Work out the finished part from the listing and answer in its coordinate system (mm). A direction names the side the tool comes from. Round coordinates to 2 decimals unless told otherwise and drop trailing zeros. Answer in a Markdown table with one row per item.
Autodesk Fusion 360 part; units mm, degrees
ref_plane "WorkPlane1" through (0, 0, 40) normal (0, 0, 1) x (1, 0, 0)
ref_plane "WorkPlane2" through (0, 0, 50) normal (0, 0, 1) x (1, 0, 0)
sketch "Sketch1" plane through (0, 0, 0) normal (0, 0, 1) x (1, 0, 0)
  line L0 (-21, 4) -> (119, 4)
  line L1 (119, 4) -> (119, 94)
  line L2 (119, 94) -> (-21, 94)
  line L3 (-21, 94) -> (-21, 4)
sketch "Sketch2" plane through (0, 0, 40) normal (0, 0, 1) x (1, 0, 0)
  line L0 (-1, -1) -> (99, -1)
  line L1 (99, -1) -> (99, 99)
  line L2 (99, 99) -> (-1, 99)
  line L3 (-1, 99) -> (-1, -1)
sketch "Sketch3" plane through (0, 0, 50) normal (0, 0, 1) x (1, 0, 0)
  line L0 (-1, -1) -> (99, -1)
  line L1 (99, -1) -> (99, 99)
  line L2 (99, 99) -> (-1, 99)
  line L3 (-1, 99) -> (-1, -1)
loft "Loft1" add profiles "Sketch1", "Sketch2", "Sketch3" section 1 section 2 section 3
sketch "Sketch4" plane through (0, 0, 0) normal (0, 0, 1) x (1, 0, 0)
  line L0 (-19, 6) -> (117, 6)
  line L1 (117, 6) -> (117, 92)
  line L2 (117, 92) -> (-19, 92)
  line L3 (-19, 92) -> (-19, 6)
sketch "Sketch5" plane through (0, 0, 40) normal (0, 0, 1) x (1, 0, 0)
  line L0 (-0.1, -0.1) -> (98.1, -0.1)
  line L1 (98.1, -0.1) -> (98.1, 98.1)
  line L2 (98.1, 98.1) -> (-0.1, 98.1)
  line L3 (-0.1, 98.1) -> (-0.1, -0.1)
sketch "Sketch6" plane through (0, 0, 50) normal (0, 0, 1) x (1, 0, 0)
  line L0 (0.2, 0.2) -> (97.8, 0.2)
  line L1 (97.8, 0.2) -> (97.8, 97.8)
  line L2 (97.8, 97.8) -> (0.2, 97.8)
  line L3 (0.2, 97.8) -> (0.2, 0.2)
loft "Loft2" cut profiles "Sketch4", "Sketch5", "Sketch6" section 1 section 2 section 3
ref_plane "WorkPlane3" through (0, 0, 12.5) normal (0, 0, 1) x (1, 0, 0)
sketch "Sketch7" plane through (0, 0, 12.5) normal (0, 0, 1) x (1, 0, 0)
  line L0 (19, -12) -> (79, -12)
  line L1 (79, -12) -> (79, 0.3)
  line L2 (79, 0.3) -> (19, 0.3)
  line L3 (19, 0.3) -> (19, -12)
extrude "Extrude1" add sketch "Sketch7" along normal blind 15
1) Find the intervals of material crossed by probe 1 along Y at (x, z) = (39, 15.5); probe 2 along Y at (x, z) = (94.5, 19); probe 3 along X at (y, z) = (27, 42), in increasing order. Write a range as from..to.
Filled in:
| item | result |
|---|---|
| probe 1 | y = -12..0.3, 0.95..2.03, 95.97..97.05 |
| probe 2 | y = 0.47..1.44, 96.56..97.53 |
| probe 3 | x = -0.87..0.08, 97.92..98.87 |
2) The mould has two halves that part along Y. Classify faces 3 (the face through (49, -12, 20)), 4 (the face through (19, -6, 20)), 5 (the face through (49, 0.3, 16)): released by +Y, released by -Y, zero draft, split by the parting line, or undercut.
Filled in:
| item | result |
|---|---|
| face 3 | released by -Y |
| face 4 | zero draft |
| face 5 | undercut |
3) Find section A-A, the plane z = 15. Give the number of separate pieces and of enclosed holes in the cut face, then the cut area to 3 significant figures.
Filled in:
| item | result |
|---|---|
| separate pieces | 2 |
| enclosed holes | 1 |
| area | 1,190 mm^2 |
4) Each of these flat-tipped pins is pushed along its axis until it touches: pin 1 (10 mm diameter, centred on x = 67.5, z = 36, fed in from +Y); pin 2 (1 mm diameter, centred on y = 43, z = 41.5, fed in from +X); pin 3 (10 mm diameter, centred on y = 33, z = 32.5, fed in from -X). Where does it stop, or does it pass through?
Filled in:
| item | result |
|---|---|
| pin 1 | stops at y = 99.02 |
| pin 2 | stops at x = 98.93 |
| pin 3 | stops at x = -3.45 |
5) Which of the six approach directions +Z, -Z, +X, -X, +Y, -Y give full straight-line access (tool end or side, diameter ignored) to faces 1 (the face through (35, 5, 0)), 2 (the face through (49, -6, 12.5))?
Filled in:
| item | result |
|---|---|
| face 1 | -Z, +X, -X, +Y, -Y |
| face 2 | -Z, +X, -X, -Y |
